from build123d import *

# Parameters (mm, degrees)
BOSS_EXTRUDE1_DEPTH          = 7.9375
FILLET1_R                    = 25.4
FILLET2_R                    = 16.51
F_3_8_CLEARANCE_HOLE1_D      = 9.8044
EXTRUDE_THIN1_DEPTH          = 7.9375
CUT_EXTRUDE_THIN2_START      = -7.9375
CUT_EXTRUDE_THIN2_DEPTH      = 7.9375
CUT_EXTRUDE_THIN1_DEPTH      = 171.11453265
CUT_EXTRUDE_THIN1_DEPTH_BACK = 152.4
FILLET4_R                    = 6.35


with BuildPart() as part:
    # Sketch1 → Boss-Extrude1 (new body)
    with BuildSketch(Plane(origin=(0, 0, 0), x_dir=(0, 0, -1), z_dir=(1, 0, 0))):
        with BuildLine():
            Line((34.925, -84.1375), (63.5, -84.1375))
            ThreePointArc((63.5, -84.1375), (147.6375, 0), (63.5, 84.1375))
            Line((63.5, 84.1375), (-63.5, 84.1375))
            ThreePointArc((-63.5, 84.1375), (-147.6375, 0), (-63.5, -84.1375))
            Line((-63.5, -84.1375), (-34.925, -84.1375))
            Line((-34.925, -84.1375), (-31.75, -74.6125))
            Line((-31.75, -74.6125), (-68.2625, -46.0375))
            Line((-68.2625, -46.0375), (-68.2625, -4.7625))
            Line((-68.2625, -4.7625), (68.2625, -4.7625))
            Line((68.2625, -4.7625), (68.2625, -46.0375))
            Line((68.2625, -46.0375), (31.75, -74.6125))
            Line((31.75, -74.6125), (34.925, -84.1375))
        make_face()
    extrude(amount=BOSS_EXTRUDE1_DEPTH)

    # Fillet1
    fillet1_edges = [part.edges().sort_by_distance(p)[0] for p in [
        (3.96875, -46.0375, -68.2625),
        (3.96875, -46.0375, 68.2625),
    ]]
    fillet(fillet1_edges, radius=FILLET1_R)

    # Fillet2
    fillet2_edges = [part.edges().sort_by_distance(p)[0] for p in [
        (3.96875, -4.7625, -68.2625),
        (3.96875, -4.7625, 68.2625),
    ]]
    fillet(fillet2_edges, radius=FILLET2_R)

    # 3/8 Clearance Hole1 (through all)
    with Locations(Plane(origin=(7.9375, 30.1625, 69.85), x_dir=(0, 0, 1), z_dir=(1, 0, 0))):
        with Locations((0, 0), (-69.85, 0), (-139.7, 0)):
            Hole(F_3_8_CLEARANCE_HOLE1_D / 2)

    # Sketch9 → Extrude-Thin1 (add)
    with BuildSketch(Plane(origin=(7.9375, 0, 0), x_dir=(0, 0, -1), z_dir=(1, 0, 0))):
        with BuildLine():
            Line((-31.75, -74.6125), (-63.217410815, -49.985830667))
            ThreePointArc((-63.217410815, -49.985830667), (-71.54294782, -21.815600163), (-47.625, -4.7625))
            Line((-47.625, -4.7625), (47.625, -4.7625))
            ThreePointArc((47.625, -4.7625), (71.54294782, -21.815600163), (63.217410815, -49.985830667))
            Line((63.217410815, -49.985830667), (31.75, -74.6125))
            Line((31.75, -74.6125), (34.880845969, -78.613025405))
            Line((34.880845969, -78.613025405), (66.348256784, -53.986356072))
            ThreePointArc((66.348256784, -53.986356072), (76.34550282, -20.159742237), (47.625, 0.3175))
            Line((47.625, 0.3175), (-47.625, 0.3175))
            ThreePointArc((-47.625, 0.3175), (-76.34550282, -20.159742237), (-66.348256784, -53.986356072))
            Line((-66.348256784, -53.986356072), (-34.880845969, -78.613025405))
            Line((-34.880845969, -78.613025405), (-31.75, -74.6125))
        make_face()
    extrude(amount=-EXTRUDE_THIN1_DEPTH)

    # Sketch9<2> → Cut-Extrude-Thin2 (cut)
    with BuildSketch(Plane(origin=(7.9375, 0, 0), x_dir=(0, 0, -1), z_dir=(1, 0, 0)).offset(CUT_EXTRUDE_THIN2_START)):
        with BuildLine():
            Line((-31.75, -74.6125), (-63.217410815, -49.985830667))
            ThreePointArc((-63.217410815, -49.985830667), (-71.54294782, -21.815600163), (-47.625, -4.7625))
            Line((-47.625, -4.7625), (47.625, -4.7625))
            ThreePointArc((47.625, -4.7625), (71.54294782, -21.815600163), (63.217410815, -49.985830667))
            Line((63.217410815, -49.985830667), (31.75, -74.6125))
            Line((31.75, -74.6125), (27.053731046, -68.611711892))
            Line((27.053731046, -68.611711892), (58.521141861, -43.985042559))
            ThreePointArc((58.521141861, -43.985042559), (64.339115319, -24.299387052), (47.625, -12.3825))
            Line((47.625, -12.3825), (-47.625, -12.3825))
            ThreePointArc((-47.625, -12.3825), (-64.339115319, -24.299387052), (-58.521141861, -43.985042559))
            Line((-58.521141861, -43.985042559), (-27.053731046, -68.611711892))
            Line((-27.053731046, -68.611711892), (-31.75, -74.6125))
        make_face()
    extrude(amount=CUT_EXTRUDE_THIN2_DEPTH, mode=Mode.SUBTRACT)

    # Sketch7 → Cut-Extrude-Thin1 (cut, two sides: drawn at the far end of the back side and taken through both)
    with BuildSketch(Plane(origin=(7.9375, 0, 0), x_dir=(0, 0, -1), z_dir=(1, 0, 0)).offset(-CUT_EXTRUDE_THIN1_DEPTH_BACK)):
        with BuildLine():
            Line((31.75, -74.6125), (44.45, -76.851852655))
            ThreePointArc((44.45, -76.851852655), (101.359893984, -56.480810426), (112.805620908, 2.871617747))
            ThreePointArc((112.805620908, 2.871617747), (86.188258708, 38.731700552), (43.668279277, 52.3875))
            Line((43.668279277, 52.3875), (-43.668279277, 52.3875))
            ThreePointArc((-43.668279277, 52.3875), (-86.188258708, 38.731700552), (-112.805620908, 2.871617747))
            ThreePointArc((-112.805620908, 2.871617747), (-101.359893984, -56.480810426), (-44.45, -76.851852655))
            Line((-44.45, -76.851852655), (-31.75, -74.6125))
            Line((-31.75, -74.6125), (-23.810805317, -119.637910468))
            Line((-23.810805317, -119.637910468), (-36.510805317, -121.877263123))
            ThreePointArc((-36.510805317, -121.877263123), (-136.068541071, -86.240316762), (-156.091608712, 17.590369727))
            ThreePointArc((-156.091608712, 17.590369727), (-112.809463221, 75.901982637), (-43.668279277, 98.1075))
            Line((-43.668279277, 98.1075), (43.668279277, 98.1075))
            ThreePointArc((43.668279277, 98.1075), (112.809463221, 75.901982637), (156.091608712, 17.590369727))
            ThreePointArc((156.091608712, 17.590369727), (136.068541071, -86.240316762), (36.510805317, -121.877263123))
            Line((36.510805317, -121.877263123), (23.810805317, -119.637910468))
            Line((23.810805317, -119.637910468), (31.75, -74.6125))
        make_face()
    extrude(amount=CUT_EXTRUDE_THIN1_DEPTH + CUT_EXTRUDE_THIN1_DEPTH_BACK, mode=Mode.SUBTRACT)

    # Fillet4
    fillet4_edges = [part.edges().sort_by_distance(p)[0] for p in [
        (3.96875, -74.6125, 31.75),
        (3.96875, -74.6125, -31.75),
    ]]
    fillet(fillet4_edges, radius=FILLET4_R)


solid = part.part
Can you work these out from the model? Positions are in its coordinate system, mm. A direction names the side the tool comes from. Coordinates: 2 decimals unless noted, no trailing zeros. Write each loop counter-clockwise with the first axis right and the second up, starting at its lowest first coordinate (ties: lowest second). Pieces come first, ordered by that corner, then holes. Notation, with made-up numbers: (32, -33.75) -> (37, -33.75) arc R14 ccw to (37, -21.75) -> close; hole circle Ø1 at (10.5, -15.75). An arc over 180 degrees is marked (long way). Answer as CSV lines item,"result".
1) Will these pins go through, and if not, where does the flat tip stop? P1, Ø4, axis at x = 1.5, z = -8, coming from the -Y side; P2, Ø2, axis at x = 6, y = -1, coming from the -Z side; P3, Ø1.5, axis at x = 1, z = 70.5, coming from the -Y side.
Check result:
P1,"y = -4.76"
P2,"z = -114.24"
P3,"y = -75.98"
2) If we section it at A-A on z = 0: Please give me the cut outline in (x, y).
Check result:
outline,"(0, -4.76) -> (7.94, -4.76) -> (7.94, 25.26) -> (0, 25.26) -> close; (0, 35.06) -> (7.94, 35.06) -> (7.94, 52.39) -> (0, 52.39) -> close"
3) On a 3-axis mill with a long thin cutter (end or side, diameter ignored), from which of +Z, -Z, +X, -X, +Y, -Y can I reach the whole of each face in a straight line? I mean faces 1 (the cylindrical face through (3.913, -21.402, -71.396)), 2 (the flat face through (7.938, 3, 2)). Say none if no direction works.
Check result:
face 1,"+X, -X"
face 2,"+Z, -Z, +X, +Y, -Y"
4) If we mould it in two halves opening along Z, with no side actions, what happens to faces 3 (the cylindrical face through (3.91, 34.95, 1.06)), 4 (the cylindrical face through (3.91, 39.1, 85.67)), 5 (the flat face through (4, 52.388, -1)), 6 (the cylindrical face through (3.91, 38.36, -86.7))? For each: +Z half, -Z half, draft (parallel to the pull), parting line (faces both ways), or undercut.
Check result:
face 3,"undercut"
face 4,"+Z half"
face 5,"draft"
face 6,"-Z half"
5) If we section it at C-C on z = -69.85: Please give me the cut outline in (x, y), then the cut area to 3 significant figures.
Check result:
outline,"(0, -75.95) -> (7.94, -75.95) -> (7.94, -42.15) -> (0, -42.15) -> close; (0, -17.97) -> (7.94, -17.97) -> (7.94, 25.26) -> (0, 25.26) -> close; (0, 35.06) -> (7.94, 35.06) -> (7.94, 47.53) -> (0, 47.53) -> close"
area,"710 mm²"
6) If we section it at D-D on x = 5.5: Count the separate pieces of the cut face and the enclosed holes in it, then the cut area to 3 significant figures.
Check result:
separate pieces,"1"
enclosed holes,"3"
area,"17,300 mm²"
7) If I drill on line 1 (Y direction, x = 4.5, z = 69.85); line 2 (Z direction, x = 1, y = 32.5); line 3 (Z direction, x = 7.75, y = -32), over which ranges is the centre line in solid material (lowest first)? Write a range as from..to.
Check result:
line 1,"-75.95..-42.15, -17.97..25.26, 35.06..47.53"
line 2,"-93.76..-74.16, -65.54..-4.31, 4.31..65.54, 74.16..93.76"
line 3,"-114.12..-72.85, 72.85..114.12"
8) If we section it at B-B on y = -24: Please give me the cut outline in (x, z), then the cut area to 3 significant figures.
Check result:
outline,"(0, -115.62) -> (7.94, -115.62) -> (7.94, -72.19) -> (0, -72.19) -> close; (0, 72.19) -> (7.94, 72.19) -> (7.94, 115.62) -> (0, 115.62) -> close"
area,"690 mm²"
